from build123d import *

# Parameters (mm, degrees)
BOSS_EXTRUDE1_DEPTH = 22.5
SKETCH2_R           = 3.6
CUT_EXTRUDE1_DEPTH  = 51
SKETCH3_R           = 3.6
CUT_EXTRUDE2_DEPTH  = 51
FILLET1_R           = 4


with BuildPart() as part:
    # Sketch1 → Boss-Extrude1 (new body)
    with BuildSketch(Plane.XY):
        Polygon((0, 50), (0, 0), (50, 0), (50, 4.5), (4.5, 4.5), (4.5, 50), align=None)
    extrude(amount=BOSS_EXTRUDE1_DEPTH)

    # Sketch2 → Cut-Extrude1 (cut, through all)
    with BuildSketch(Plane.ZY):
        with Locations((11.25, 37.5)):
            Circle(SKETCH2_R)
        with Locations((11.25, 12.5)):
            Circle(SKETCH2_R)
    extrude(amount=-CUT_EXTRUDE1_DEPTH, mode=Mode.SUBTRACT)

    # Sketch3 → Cut-Extrude2 (cut, through all)
    with BuildSketch(Plane.XZ):
        with Locations((37.5, 11.25)):
            Circle(SKETCH3_R)
        with Locations((12.5, 11.25)):
            Circle(SKETCH3_R)
    extrude(amount=-CUT_EXTRUDE2_DEPTH, mode=Mode.SUBTRACT)

    # Fillet1
    fillet1_edges = [part.edges().sort_by_distance(p)[0] for p in [
        (4.5, 50, 11.25),
        (50, 4.5, 11.25),
    ]]
    fillet(fillet1_edges, radius=FILLET1_R)


solid = part.part
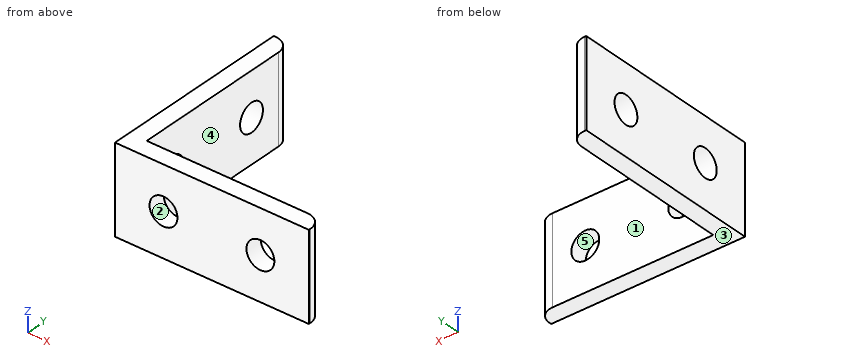
Could you check a few things on this model? Use its own coordinates, in mm. Face numbers are marked on the shaded views. A direction names the side the tool comes from. Give positions to 0.01 mm unless a question says otherwise; leave off trailing zeros. Order: outer loops, then holes, each group sorted by start corner. A loop starts at its lowest first (then second) coordinate and runs counter-clockwise, first axis right, second up. Notation, with made-up numbers: (-8.75, 50) -> (18.25, 50) arc R27 ccw to (18.25, 86) -> close; hole circle Ø2 at (86.5, 45.25). An arc over 180 degrees is marked (long way). Return JSON: item names as keys, results as strings.
1. For pin 1 Ø1.5 at (y, z) = (17.5, 19.5) entering from +X; pin 2 Ø6 at (x, z) = (42.5, 15) entering from +Y, each with a flat end and sliding along its axis, tell me the tip position at first contact or that it passes through.
Answer list:
{"pin 1": "stops at x = 4.5", "pin 2": "stops at y = 4.5"}
2. Imagine slicing it at A-A on x = 12.5. List the corners of the cut face in (y, z) for me.
Answer list:
{"outline": "(0, 0) -> (4.5, 0) -> (4.5, 7.65) -> (0, 7.65) -> close; (0, 14.85) -> (4.5, 14.85) -> (4.5, 22.5) -> (0, 22.5) -> close"}
3. On a 3-axis mill with a long thin cutter (end or side, diameter ignored), from which of +Z, -Z, +X, -X, +Y, -Y can I reach the whole of each face in a straight line? I mean the marked faces 1 and 2. Say none if no direction works.
Answer list:
{"face 1": "+Z, -Z, +X, +Y", "face 2": "+Y, -Y"}
4. I need wall thicknesses on line 1 (Y direction, x = 1.35, z = 11.25); line 2 (X direction, y = 21, z = 9.5). Which ranges of each line are inside material? Lowest first, please. Write a range as from..to.
Answer list:
{"line 1": "y = 0..8.9, 16.1..33.9, 41.1..49.91", "line 2": "x = 0..4.5"}
5. Thinking about a two-plate mould opening in Z: for the marked faces 3, 4 and 5, which applies, pulls with the +Z half, pulls with the -Z half, needs draft (parallel to the pull), parting line crosses it, or undercut?
Answer list:
{"face 3": "pulls with the -Z half", "face 4": "needs draft", "face 5": "undercut"}
6. Imagine slicing it at C-C on z = 11.25. List the corners of the cut face in (x, y) for me.
Answer list:
{"outline": "(0, 0) -> (8.9, 0) -> (8.9, 4.5) -> (4.5, 4.5) -> (4.5, 8.9) -> (0, 8.9) -> close; (0, 16.1) -> (4.5, 16.1) -> (4.5, 33.9) -> (0, 33.9) -> close; (0, 41.1) -> (4.5, 41.1) -> (4.5, 46) arc R4 ccw to (0.5, 50) -> (0, 50) -> close; (16.1, 0) -> (33.9, 0) -> (33.9, 4.5) -> (16.1, 4.5) -> close; (41.1, 0) -> (50, 0) -> (50, 0.5) arc R4 ccw to (46, 4.5) -> (41.1, 4.5) -> close"}
7. Imagine slicing it at D-D on z = 19.25. List the corners of the cut face in (x, y) for me, then the cut area to 3 significant figures.
Answer list:
{"outline": "(0, 0) -> (50, 0) -> (50, 0.5) arc R4 ccw to (46, 4.5) -> (4.5, 4.5) -> (4.5, 46) arc R4 ccw to (0.5, 50) -> (0, 50) -> close", "area": "423 mm2"}
